Model file for the job. Use its own axes, mm. Coordinates: 2 decimals unless noted, no trailing zeros. Return JSON: item names as keys, results as strings. Group by question number.
1) Cut at A-A (z = 16). State how many separate pieces and enclosed holes the cut face has, and give its area (3 significant figures).
2) Flat gauge pin, fed straight in: pin 1 (1.5 mm diameter, centred on x = -47.5, y = 0.5, fed in from -Z). Where does the tip first touch, or does it go through?
3) Probe line 1 (Z direction, x = 9, y = 3.5); line 2 (X direction, y = 8.75, z = -97); line 3 (X direction, y = -7, z = 98). List the from-to ranges inside material, lowest first.
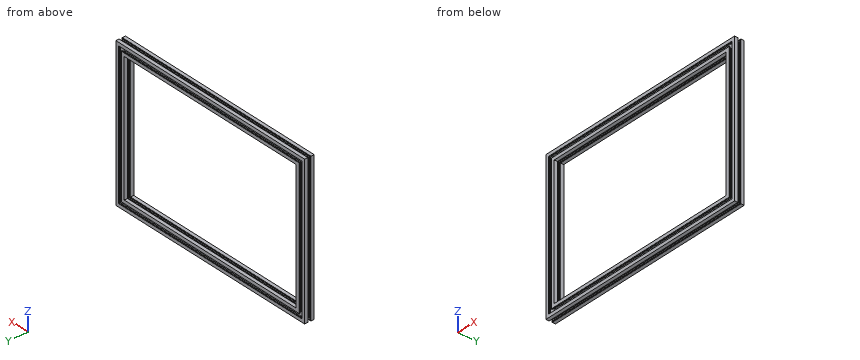
from build123d import *

# Parameters (mm, degrees)
CROQUIS2_R = 2.5


with BuildPart() as part:
    # Barrer1: sweep along a path in Croquis1
    with BuildLine(Plane(origin=(0, 0, 0), x_dir=(1, 0, 0), z_dir=(0, 1, 0))) as barrer1_path:
        Line((-210.93, 141.5), (210.93, 141.5))
        Line((210.93, 141.5), (210.93, -141.5))
        Line((210.93, -141.5), (-210.93, -141.5))
        Line((-210.93, -141.5), (-210.93, 141.5))
    # Croquis2 → Barrer1 (sweep)
    with BuildSketch(Plane(origin=(0, 0, 0), x_dir=(0, 0, -1), z_dir=(1, 0, 0))):
        Polygon((-144.848190044, 9.751218458), (-144.848190044, 9.391218458), (-144.343190044, 9.391218458), (-144.343190044, 8.021218458), (-146.678190044, 8.021218458), (-146.678190044, 6.721218458), (-145.121709911, 5.163799744), (-137.875239336, 5.163799744), (-136.318759202, 6.721218458), (-136.318759202, 8.021218458), (-138.653759202, 8.021218458), (-138.653759202, 9.391218458), (-138.148759202, 9.391218458), (-138.148759202, 9.751218458), (-131.747639801, 9.751218458), (-131.747639801, 3.185976388), (-132.107639736, 3.185759368), (-132.107335305, 2.68075946), (-133.477335056, 2.679933578), (-133.478742672, 5.014933154), (-134.778742435, 5.01414947), (-136.335222569, 3.456730756), (-136.335222569, -3.455477102), (-134.778742435, -5.012895817), (-133.478742672, -5.0136795), (-133.477335056, -2.678679924), (-132.107335305, -2.679505806), (-132.107639736, -3.184505714), (-131.747639801, -3.184722734), (-131.747639801, -9.749964804), (-138.148759202, -9.749964804), (-138.148759202, -9.389964804), (-138.653759202, -9.389964804), (-138.653759202, -8.019964804), (-136.318759202, -8.019964804), (-136.318759202, -6.719964804), (-137.875239336, -5.16254609), (-145.121709911, -5.16254609), (-146.678190044, -6.719964804), (-146.678190044, -8.019964804), (-144.343190044, -8.019964804), (-144.343190044, -9.389964804), (-144.848190044, -9.389964804), (-144.848190044, -9.749964804), (-151.249309446, -9.749964804), (-151.249309446, -3.184722734), (-150.889309511, -3.184505714), (-150.889613942, -2.679505806), (-149.519614191, -2.678679924), (-149.518206575, -5.0136795), (-148.218206811, -5.012895817), (-146.661726678, -3.455477102), (-146.661726678, 3.456730756), (-148.218206811, 5.01414947), (-149.518206575, 5.014933154), (-149.519614191, 2.679933578), (-150.889613942, 2.68075946), (-150.889309511, 3.185759368), (-151.249309446, 3.185976388), (-151.249309446, 9.751218458), align=None)
        with Locations((-141.498474623, 0.000626827)):
            Circle(CROQUIS2_R, mode=Mode.SUBTRACT)
    sweep(path=barrer1_path.line, transition=Transition.RIGHT)


solid = part.part
Answers below:
{
 "1": {"separate pieces": "2", "enclosed holes": "2", "area": "428 mm^2"},
 "2": {"pin 1": "stops at z = -146.66"},
 "3": {"line 1": "z = -151.25 to -149.52, -146.7 to -136.29, -133.48 to -131.75, 131.75 to 133.48, 136.29 to 146.7, 149.52 to 151.25", "line 2": "x = -220.68 to -213.77, -208.08 to -201.18, 201.18 to 208.08, 213.77 to 220.68", "line 3": "x = -220.68 to -216.11, -205.75 to -201.18, 201.18 to 205.75, 216.11 to 220.68"}
}
